Here's how the part is built. I have some questions about the finished solid (model axes, mm). A direction names the side the tool comes from. Coordinates: 2 decimals unless noted, no trailing zeros. Write each loop counter-clockwise with the first axis right and the second up, starting at its lowest first coordinate (ties: lowest second). Pieces come first, ordered by that corner, then holes.
(1) For pin 1 Ø2.5 at (x, y) = (65, -4.5) entering from +Z; pin 2 Ø1.5 at (x, z) = (62.5, 12) entering from -Y; pin 3 Ø0.9 at (y, z) = (-4, 49.5) entering from +X, each with a flat end and sliding along its axis, tell me the tip position at first contact or that it passes through.
(2) Which directions (+Z, -Z, +X, -X, +Y, -Y) give clear straight access to the entire face, cutting with the end or side of a thin tool? Please do faces 1 (the flat face through (23, 0, 41.999)), 2 (the flat face through (68.538, -3, 65)), 3 (the flat face through (66, -5, 71.999)), 4 (the flat face through (63.538, -3, 65)).
(3) Please list where these lines run through material, in increasing order: probe 1 along X at (y, z) = (2.5, 47); probe 2 along Z at (x, y) = (26, 2.25); probe 3 along Z at (x, y) = (46, -3).
(4) Thinking about a two-plate mould opening in Z: for faces 5 (the cylindrical face through (4.139, 2.465, 18.907)), 6 (the flat face through (23, 2, 76.999)), 7 (the flat face through (-26.462, 2, 28)), which applies, released by +Z, released by -Z, zero draft, split by the parting line, or undercut?
(5) Imagine slicing it at C-C, the plane z = 33. List the corners of the cut face in (x, y) for me, plus the area to 3 significant figures.
```python
from build123d import *

# Parameters (mm, degrees)
SKETCH1_W           = 100
SKETCH1_H           = 100
SKETCH1_R           = 2
SKETCH1_W_2         = 58
SKETCH1_H_2         = 30
BOSS_EXTRUDE1_DEPTH = 5
SKETCH2_W           = 64
SKETCH2_H           = 36
SKETCH2_W_2         = 58
SKETCH2_H_2         = 30
BOSS_EXTRUDE2_DEPTH = 5
SKETCH3_W           = 64
SKETCH3_H           = 36
SKETCH3_W_2         = 52
SKETCH3_H_2         = 24
BOSS_EXTRUDE3_DEPTH = 2
FILLET2_R           = 2
SKETCH5_W           = 5
SKETCH5_H           = 10
BOSS_EXTRUDE4_DEPTH = 10
SKETCH6_R           = 2.5
CUT_EXTRUDE2_DEPTH  = 8
SKETCH7_R           = 2.5
CUT_EXTRUDE3_DEPTH  = 8


with BuildPart() as part:
    # Sketch1 → Boss-Extrude1 (new body)
    with BuildSketch(Plane(origin=(0, 0, 0), x_dir=(1, 0, 0), z_dir=(0, 1, 0))):
        with Locations((23.538461538, -26.998952175)):
            Rectangle(SKETCH1_W, SKETCH1_H)
        with Locations(Location((3.538461538, 15.001047825, 0), (0, 0, 270))):
            Circle(SKETCH1_R, mode=Mode.SUBTRACT)
        with Locations(Location((3.538461538, 7.001047825, 0), (0, 0, 270))):
            Circle(SKETCH1_R, mode=Mode.SUBTRACT)
        with Locations(Location((3.538461538, -0.998952175, 0), (0, 0, 270))):
            Circle(SKETCH1_R, mode=Mode.SUBTRACT)
        with Locations(Location((3.538461538, -8.998952175, 0), (0, 0, 270))):
            Circle(SKETCH1_R, mode=Mode.SUBTRACT)
        with Locations(Location((3.538461538, -16.998952175, 0), (0, 0, 270))):
            Circle(SKETCH1_R, mode=Mode.SUBTRACT)
        with Locations(Location((3.538461538, -24.998952175, 0), (0, 0, 270))):
            Circle(SKETCH1_R, mode=Mode.SUBTRACT)
        with Locations(Location((43.538461538, -24.998952175, 0), (0, 0, 90))):
            Circle(SKETCH1_R, mode=Mode.SUBTRACT)
        with Locations(Location((43.538461538, -16.998952175, 0), (0, 0, 90))):
            Circle(SKETCH1_R, mode=Mode.SUBTRACT)
        with Locations(Location((43.538461538, -8.998952175, 0), (0, 0, 90))):
            Circle(SKETCH1_R, mode=Mode.SUBTRACT)
        with Locations(Location((43.538461538, -0.998952175, 0), (0, 0, 90))):
            Circle(SKETCH1_R, mode=Mode.SUBTRACT)
        with Locations(Location((43.538461538, 7.001047825, 0), (0, 0, 90))):
            Circle(SKETCH1_R, mode=Mode.SUBTRACT)
        with Locations(Location((43.538461538, 15.001047825, 0), (0, 0, 90))):
            Circle(SKETCH1_R, mode=Mode.SUBTRACT)
        with Locations((23.538461538, -56.998952175)):
            Rectangle(SKETCH1_W_2, SKETCH1_H_2, mode=Mode.SUBTRACT)
    extrude(amount=BOSS_EXTRUDE1_DEPTH)

    # Sketch2 → Boss-Extrude2 (add)
    with BuildSketch(Plane.XZ):
        with Locations((23.538461538, 56.998952175)):
            Rectangle(SKETCH2_W, SKETCH2_H)
        with Locations((23.538461538, 56.998952175)):
            Rectangle(SKETCH2_W_2, SKETCH2_H_2, mode=Mode.SUBTRACT)
    extrude(amount=BOSS_EXTRUDE2_DEPTH)

    # Sketch3 → Boss-Extrude3 (add)
    with BuildSketch(Plane.XZ.offset(5)):
        with Locations((23.538461538, 56.998952175)):
            Rectangle(SKETCH3_W, SKETCH3_H)
        with Locations((23.538461538, 56.998952175)):
            Rectangle(SKETCH3_W_2, SKETCH3_H_2, mode=Mode.SUBTRACT)
    extrude(amount=BOSS_EXTRUDE3_DEPTH)

    # Fillet2
    fillet2_edges = [part.edges().sort_by_distance(p)[0] for p in [
        (49.538461538, -7, 56.998952175),
        (23.538461538, -7, 68.998952175),
        (-2.461538462, -7, 56.998952175),
        (23.538461538, -7, 44.998952175),
        (23.538461538, -7, 74.998952175),
        (55.538461538, -7, 56.998952175),
        (23.538461538, -7, 38.998952175),
        (-8.461538462, -7, 56.998952175),
        (-8.461538462, -3.5, 38.998952175),
        (55.538461538, -3.5, 38.998952175),
        (55.538461538, -3.5, 74.998952175),
        (-8.461538462, -3.5, 74.998952175),
        (-8.461538462, 0, 56.998952175),
        (23.538461538, 0, 74.998952175),
        (55.538461538, 0, 56.998952175),
        (23.538461538, 0, 38.998952175),
    ]]
    fillet(fillet2_edges, radius=FILLET2_R - 0.0001)  # a hair under: the kernel refuses the full size

    # Sketch5 → Boss-Extrude4 (add)
    with BuildSketch(Plane.XZ):
        with Locations((66.038461538, 66.998952175)):
            Rectangle(SKETCH5_W, SKETCH5_H)
    extrude(amount=BOSS_EXTRUDE4_DEPTH)

    # Sketch6 → Cut-Extrude2 (cut)
    with BuildSketch(Plane(origin=(68.538461538, 0, 0), x_dir=(0, 0, -1), z_dir=(1, 0, 0))):
        with Locations((-66.998952175, -5)):
            Circle(SKETCH6_R)
    extrude(amount=-CUT_EXTRUDE2_DEPTH, mode=Mode.SUBTRACT)

    # Sketch7 → Cut-Extrude3 (cut)
    with BuildSketch(Plane.XZ):
        with Locations(Location((-16.461538462, -13.001047825, 0), (0, 0, 270))):
            Circle(SKETCH7_R)
    extrude(amount=-CUT_EXTRUDE3_DEPTH, mode=Mode.SUBTRACT)


solid = part.part
```
Recorded:
1. pin 1: stops at z = 72
1. pin 2: stops at y = 0
1. pin 3: stops at x = 55.54
2. face 1: +Y
2. face 2: +Z, -Z, +X, -Y
2. face 3: +Z, +X, -Y
2. face 4: +Z, -Z, -Y
3. probe 1: x = -26.46 to -5.46, 52.54 to 73.54
3. probe 2: z = -23 to 42, 72 to 77
3. probe 3: z = 39 to 42, 72 to 75
4. face 5: undercut
4. face 6: released by +Z
4. face 7: zero draft
5. outline: (-26.46, 0) - (73.54, 0) - (73.54, 5) - (-26.46, 5) - close
5. area: 500 mm2
